from build123d import *

# Parameters (mm, degrees)
SKETCH14_R           = 11
BOSS_EXTRUDE7_DEPTH  = 36.75
SKETCH18_W           = 7.62
SKETCH18_H           = 4.5
BOSS_EXTRUDE9_DEPTH  = 45.94
CUT_EXTRUDE16_REACH  = 87.359
LPATTERN1_COUNT      = 17
LPATTERN1_PITCH      = 2.7
BOSS_EXTRUDE10_DEPTH = 45.94
CHAMFER2_SIZE        = 1.5
CHAMFER2_SIZE2       = 1.21467605
BOSS_EXTRUDE11_DEPTH = 45.94
BOSS_EXTRUDE12_DEPTH = 2.5
BOSS_EXTRUDE14_START = -35
BOSS_EXTRUDE14_DEPTH = 35
FILLET2_R            = 0.5


with BuildPart() as part:
    # Sketch14 → Boss-Extrude7 (new body)
    with BuildSketch(Plane.XY):
        with Locations((-43.416294802, -3.957587863)):
            Circle(SKETCH14_R)
    extrude(amount=-BOSS_EXTRUDE7_DEPTH)

    # Sketch18 → Boss-Extrude9 (add)
    with BuildSketch(Plane(origin=(0, 0, -36.75), x_dir=(-1, 0, 0), z_dir=(0, 0, -1))):
        with Locations((43.416294802, 4.092412137)):
            Rectangle(SKETCH18_W, SKETCH18_H)
    extrude(amount=BOSS_EXTRUDE9_DEPTH)

    # Sketch19 → Cut-Extrude16 (cut, up to next)
    with BuildSketch(Plane.ZY.offset(47.409754566), mode=Mode.PRIVATE) as cut_extrude16_sk1:
        with BuildLine():
            Line((-81.573331938, 3.757468407), (-80.99640478, 3.757468407))
            ThreePointArc((-80.99640478, 3.757468407), (-80.773630162, 3.685551679), (-80.634956444, 3.496951186))
            Line((-80.634956444, 3.496951186), (-80.052462184, 1.749468407))
            Line((-80.052462184, 1.749468407), (-82.517274534, 1.749468407))
            Line((-82.517274534, 1.749468407), (-81.934780275, 3.496951186))
            ThreePointArc((-81.934780275, 3.496951186), (-81.796106557, 3.685551679), (-81.573331938, 3.757468407))
        make_face()
    cut_extrude16_tool1 = extrude(cut_extrude16_sk1.sketch, amount=-CUT_EXTRUDE16_REACH, mode=Mode.PRIVATE) & part.part
    cut_extrude16 = cut_extrude16_tool1.solids().sort_by_distance((-47.409755, 2.620329, -81.284868))[0]
    add(cut_extrude16, mode=Mode.SUBTRACT)

    # LPattern1: Cut-Extrude16 ×17
    with Locations(*[(0, 0, i * LPATTERN1_PITCH) for i in range(1, LPATTERN1_COUNT)]):
        add(cut_extrude16, mode=Mode.SUBTRACT)

    # Sketch20 → Boss-Extrude10 (add)
    with BuildSketch(Plane(origin=(0, 0, -36.75), x_dir=(-1, 0, 0), z_dir=(0, 0, -1))):
        with BuildLine():
            Line((39.606294802, 6.342412137), (47.226294802, 6.342412137))
            Line((47.226294802, 6.342412137), (47.226294802, 6.36151578))
            ThreePointArc((47.226294802, 6.36151578), (43.416294802, 7.042412137), (39.606294802, 6.36151578))
            Line((39.606294802, 6.36151578), (39.606294802, 6.342412137))
        make_face()
    extrude(amount=BOSS_EXTRUDE10_DEPTH)

    # Chamfer1: read off the stored shape, not the designer's step
    # Chamfer1 outline → Chamfer1 (revolve, cut)
    with BuildSketch(Plane(origin=(-43.416294802, -3.957587863, 0), x_dir=(1, 0, 0), z_dir=(0, -1, 0))):
        Polygon((11.000000059, -82.589999941), (10.9, -82.69), (11.000000059, -82.69), align=None)
    revolve(axis=Axis((-43.416294802, -3.957587863, 0), (0, 0, 1)), mode=Mode.SUBTRACT)

    # Chamfer2
    chamfer2_edges = [part.edges().sort_by_distance(p)[0] for p in [
        (-54.416294802, -3.957587863, 0),
    ]]
    chamfer2_side = [part.faces().sort_by_distance(p)[0] for p in [
        (-54.416294802, -3.957587863, -18.375),
    ]]
    chamfer(chamfer2_edges, length=CHAMFER2_SIZE, length2=CHAMFER2_SIZE2, reference=chamfer2_side[0])

    # Sketch21 → Boss-Extrude11 (add)
    with BuildSketch(Plane(origin=(0, 0, -36.75), x_dir=(-1, 0, 0), z_dir=(0, 0, -1))):
        with BuildLine():
            Line((39.606294802, 1.842412137), (39.606294802, 6.36151578))
            ThreePointArc((39.606294802, 6.36151578), (36.46072284, 4.564150146), (34.069637646, 1.842412137))
            Line((34.069637646, 1.842412137), (39.606294802, 1.842412137))
        make_face()
    extrude(amount=BOSS_EXTRUDE11_DEPTH)

    # Sketch23 → Boss-Extrude12 (add)
    with BuildSketch(Plane.XZ.offset(-1.842412137)):
        Polygon((-39.606294802, -36.883443427), (-39.606294802, -36.75), (-34.069637646, -36.75), (-34.069637646, -82.69), (-39.606294802, -82.69), (-39.606294802, -82.486293291), align=None)
    extrude(amount=BOSS_EXTRUDE12_DEPTH)

    # Chamfer4: read off the stored shape, not the designer's step
    # Chamfer4 outline → Chamfer4 (revolve, cut)
    with BuildSketch(Plane(origin=(-43.416294802, -3.957587863, 0), x_dir=(1, 0, 0), z_dir=(0, -1, 0))):
        Polygon((7.999999773, -82.690000227), (11.000000044, -82.69000017), (11.000000035, -79.69), align=None)
    revolve(axis=Axis((-43.416294802, -3.957587863, 0), (0, 0, 1)), mode=Mode.SUBTRACT)

    # Sketch24 → Boss-Extrude14 (add)
    with BuildSketch(Plane(origin=(0, 0, -36.75), x_dir=(-1, 0, 0), z_dir=(0, 0, -1)).offset(BOSS_EXTRUDE14_START)):
        with BuildLine():
            Line((42.666294802, 7.016814171), (42.666294802, 8.292412137))
            Line((42.666294802, 8.292412137), (44.166294802, 8.292412137))
            Line((44.166294802, 8.292412137), (44.166294802, 7.016814171))
            ThreePointArc((44.166294802, 7.016814171), (43.416294802, 7.042412137), (42.666294802, 7.016814171))
        make_face()
    extrude(amount=BOSS_EXTRUDE14_DEPTH)

    # Fillet2
    fillet2_edges = [part.edges().sort_by_distance(p)[0] for p in [
        (-42.666294802, 8.292412137, -19.25),
        (-44.166294802, 8.292412137, -19.25),
    ]]
    fillet(fillet2_edges, radius=FILLET2_R)


solid = part.part
Here's how the part is built. I have some questions about the finished solid (model axes, mm). Give positions to 0.01 mm unless a question says otherwise; leave off trailing zeros. Order: outer loops, then holes, each group sorted by start corner. A loop starts at its lowest first (then second) coordinate and runs counter-clockwise, first axis right, second up. Notation, with made-up numbers: (62, -22) -> (78, -22) arc R23 ccw to (78, 9) -> close; hole circle Ø10 at (54.5, 1.25). An arc over 180 degrees is marked (long way). Use a Markdown table: item, result. Add a question column.
Item 1: I need wall thicknesses on line 1 (Z direction, x = -42.25, y = -5.5); line 2 (X direction, y = 0.75, z = -49); line 3 (X direction, y = 3.25, z = -33). Which ranges of each line are inside material? Lowest first, please.
Item 2: Will these pins go through, and if not, where does the flat tip stop? pin 1 (2 mm diameter, centred on x = -35.5, z = -9, fed in from -Y); pin 2 (1.3 mm diameter, centred on y = 1, z = -58, fed in from +X); pin 3 (3 mm diameter, centred on y = -1, z = -32.5, fed in from +X); pin 4 (10 mm diameter, centred on y = -10, z = -52.5, fed in from -X).
Item 3: If we mould it in two halves opening along Z, with no side actions, what happens to faces 1 (the face through (-43.47, 2.681, -47.963)), 2 (the face through (-37, -0.658, -59)), 3 (the face through (-43.47, 2.681, -64.163))? For each: pulls with the +Z half, pulls with the -Z half, needs draft (parallel to the pull), parting line crosses it, or undercut.
Item 4: Imagine slicing it at A-A on z = -26.5. Please give me the cut outline in (x, y).
Data:
| question | item | result |
|---|---|---|
| 1 | line 1 | z = -36.75 to 0 |
| 1 | line 2 | x = -39.61 to -34.07 |
| 1 | line 3 | x = -51.73 to -35.11 |
| 2 | pin 1 | stops at y = -12.51 |
| 2 | pin 2 | stops at x = -34.07 |
| 2 | pin 3 | stops at x = -32.51 |
| 2 | pin 4 | passes through |
| 3 | face 1 | undercut |
| 3 | face 2 | needs draft |
| 3 | face 3 | undercut |
| 4 | outline | (-44.17, 7.02) arc R11 ccw (long way) to (-42.67, 7.02) -> (-42.67, 7.79) arc R0.5 ccw to (-43.17, 8.29) -> (-43.67, 8.29) arc R0.5 ccw to (-44.17, 7.79) -> close |
